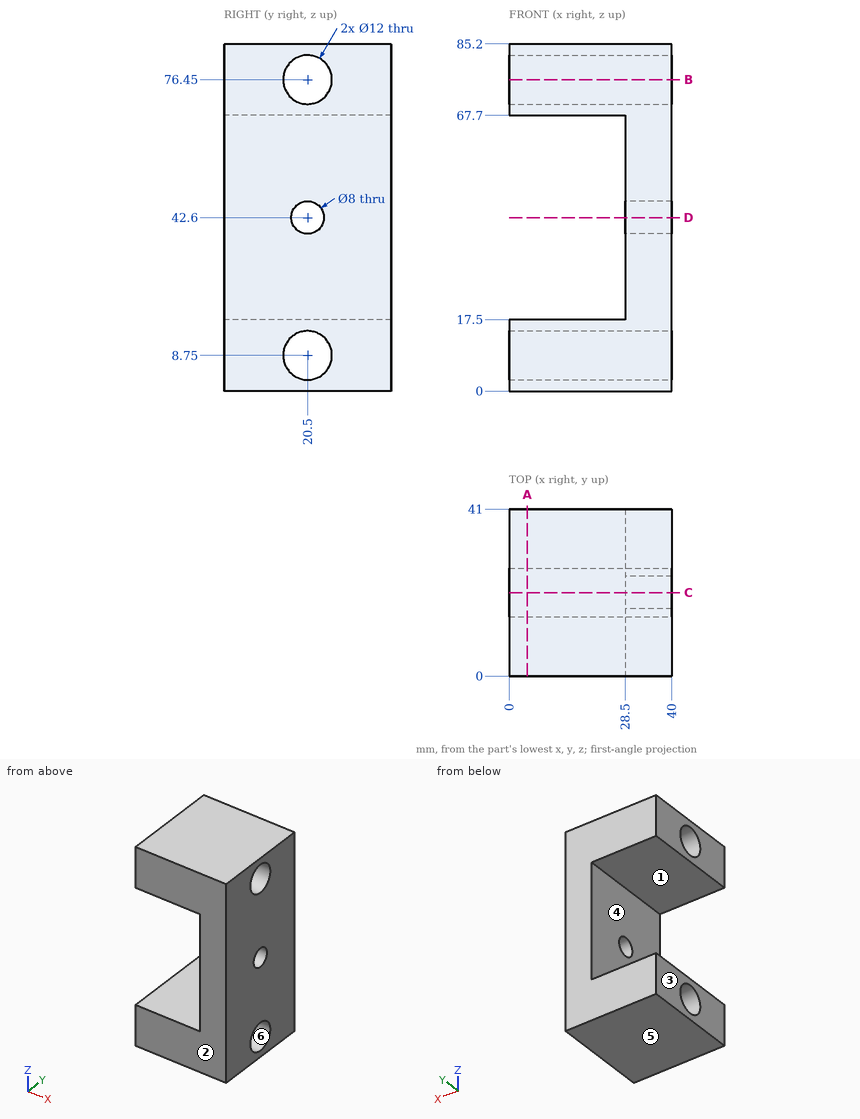
Verification items for this drawing (mm, ordinates from the low corner). A direction names the side the tool comes from. Coordinates: 2 decimals unless noted, no trailing zeros. Write each loop counter-clockwise with the first axis right and the second up, starting at its lowest first coordinate (ties: lowest second). Pieces come first, ordered by that corner, then holes. Notation, with made-up numbers: M 34.5,-7.5 L 66.5,-7.5 A22 cw 66.5,13.5 Z; hole C 35.25,50.25 d8. An arc over 180 degrees is marked long. One line per item, written item: value. Start each with the question number.
(1) Tool access check on the marked faces 1 and 2. Record the directions out of +Z, -Z, +X, -X, +Y, -Y that give a thin tool (end or side, any length) a straight path to the whole face; none if there is none.
(2) Depth check by flat-ended pin: pin 1 (6 mm diameter, centred on y = 17, z = 30, fed in from -X). Enter the tip coordinate at first touch or a pass-through.
(3) Sectioned sample at A-A, the plane x = 4.5. Enter the section's corners in (y, z), and give its area (3 significant figures).
(4) Sectioned sample at C-C, the plane y = 20.5. Enter the section's corners in (x, z).
(5) Scan lines: line 1 along Z through (x, y) = (16, 20); line 2 along Z through (x, y) = (18.5, 29.5); line 3 along Z through (x, y) = (35.5, 18). Record each from-to range of solid material in increasing order. Write a range as [from, to].
(6) Release check for a two-part mould opening along Z. For the marked faces 3, 4, 5 and 6 record: released by +Z, released by -Z, zero draft, split by the parting line, or undercut.
(7) Sectioned sample at B-B, the plane z = 76.45. Enter the section's corners in (x, y).
(8) Sectioned sample at D-D, the plane z = 42.6. Enter the section's corners in (x, y), and give its area (4 significant figures).
Filled sheet:
1. face 1: -X, +Y, -Y
1. face 2: +Z, -Z, +X, -X, -Y
2. pin 1: x = 28.5
3. outline: M 0,0 L 41,0 L 41,17.5 L 0,17.5 Z; M 0,67.7 L 41,67.7 L 41,85.2 L 0,85.2 Z; hole C 20.5,8.75 d12; hole C 20.5,76.45 d12
3. area: 1,210 mm²
4. outline: M 0,0 L 40,0 L 40,2.75 L 0,2.75 Z; M 0,14.75 L 40,14.75 L 40,38.6 L 28.5,38.6 L 28.5,17.5 L 0,17.5 Z; M 0,67.7 L 28.5,67.7 L 28.5,46.6 L 40,46.6 L 40,70.45 L 0,70.45 Z; M 0,82.45 L 40,82.45 L 40,85.2 L 0,85.2 Z
5. line 1: [0, 2.77], [14.73, 17.5], [67.7, 70.47], [82.43, 85.2]
5. line 2: [0, 17.5], [67.7, 85.2]
5. line 3: [0, 3.3], [14.2, 39.48], [45.72, 71], [81.9, 85.2]
6. face 3: zero draft
6. face 4: undercut
6. face 5: released by -Z
6. face 6: undercut
7. outline: M 0,0 L 40,0 L 40,14.5 L 0,14.5 Z; M 0,26.5 L 40,26.5 L 40,41 L 0,41 Z
8. outline: M 28.5,0 L 40,0 L 40,16.5 L 28.5,16.5 Z; M 28.5,24.5 L 40,24.5 L 40,41 L 28.5,41 Z
8. area: 379.5 mm²
